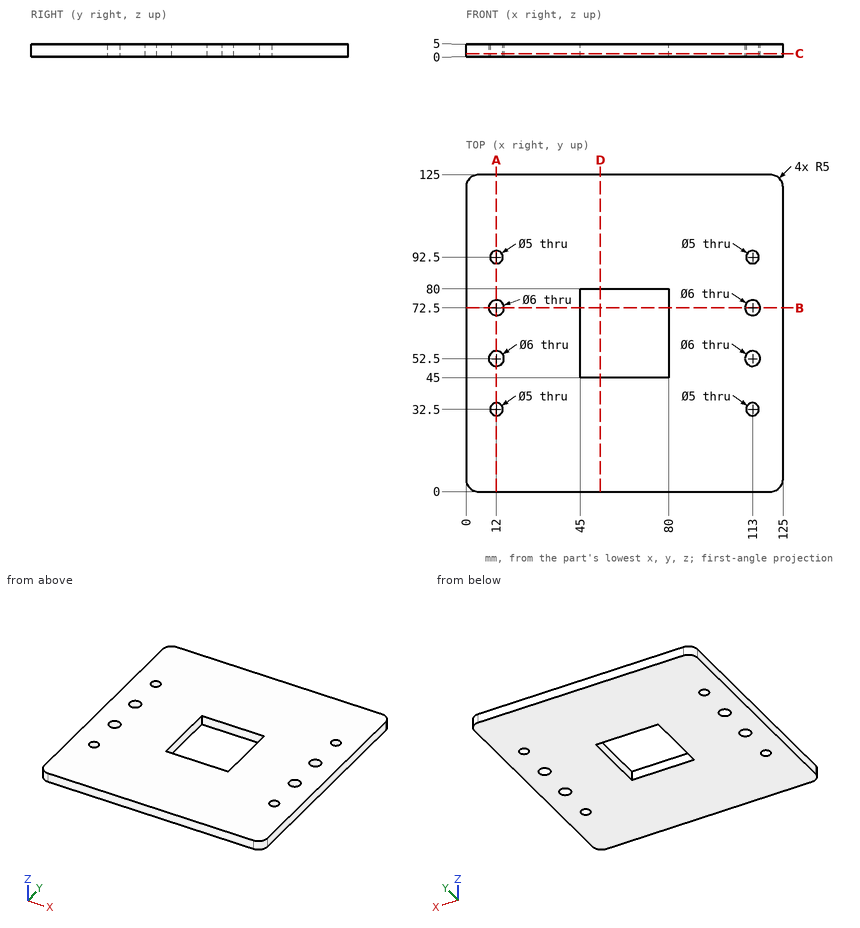
Could you check a few things on this drawing? It's one solid part, dimensions in mm from its lowest x, y, z. Coordinates: 2 decimals unless noted, no trailing zeros. Order: outer loops, then holes, each group sorted by start corner. A loop starts at its lowest first (then second) coordinate and runs counter-clockwise, first axis right, second up.
1) Imagine slicing it at A-A on x = 12. List the corners of the cut face in (y, z) for me.
2) Imagine slicing it at B-B on y = 72.5. List the corners of the cut face in (x, z) for me.
3) Imagine slicing it at D-D on x = 53. List the corners of the cut face in (y, z) for me, and give its area (3 significant figures).
4) Imagine slicing it at C-C on z = 1.2. State how many separate pieces and enclosed holes the cut face has, and give its area (3 significant figures).
5) Will this pin go through, and if not, where does the flat tip stop? pin 1 (5 mm diameter, centred on x = 113, y = 52.5, fed in from +Z).
6) I need wall thicknesses on line 1 (X direction, y = 72.5, z = 1.4); line 2 (Y direction, x = 12, z = 1.35); line 3 (X direction, y = 63.5, z = 0.6). Which ranges of each line are inside material? Lowest first, please.
Response values:
1. outline: (0, 0) - (30, 0) - (30, 5) - (0, 5) - close; (35, 0) - (49.5, 0) - (49.5, 5) - (35, 5) - close; (55.5, 0) - (69.5, 0) - (69.5, 5) - (55.5, 5) - close; (75.5, 0) - (90, 0) - (90, 5) - (75.5, 5) - close; (95, 0) - (125, 0) - (125, 5) - (95, 5) - close
2. outline: (0, 0) - (9, 0) - (9, 5) - (0, 5) - close; (15, 0) - (45, 0) - (45, 5) - (15, 5) - close; (80, 0) - (110, 0) - (110, 5) - (80, 5) - close; (116, 0) - (125, 0) - (125, 5) - (116, 5) - close
3. outline: (0, 0) - (45, 0) - (45, 5) - (0, 5) - close; (80, 0) - (125, 0) - (125, 5) - (80, 5) - close
3. area: 450 mm2
4. separate pieces: 1
4. enclosed holes: 9
4. area: 14,200 mm2
5. pin 1: passes through
6. line 1: x = 0 to 9, 15 to 45, 80 to 110, 116 to 125
6. line 2: y = 0 to 30, 35 to 49.5, 55.5 to 69.5, 75.5 to 90, 95 to 125
6. line 3: x = 0 to 45, 80 to 125
